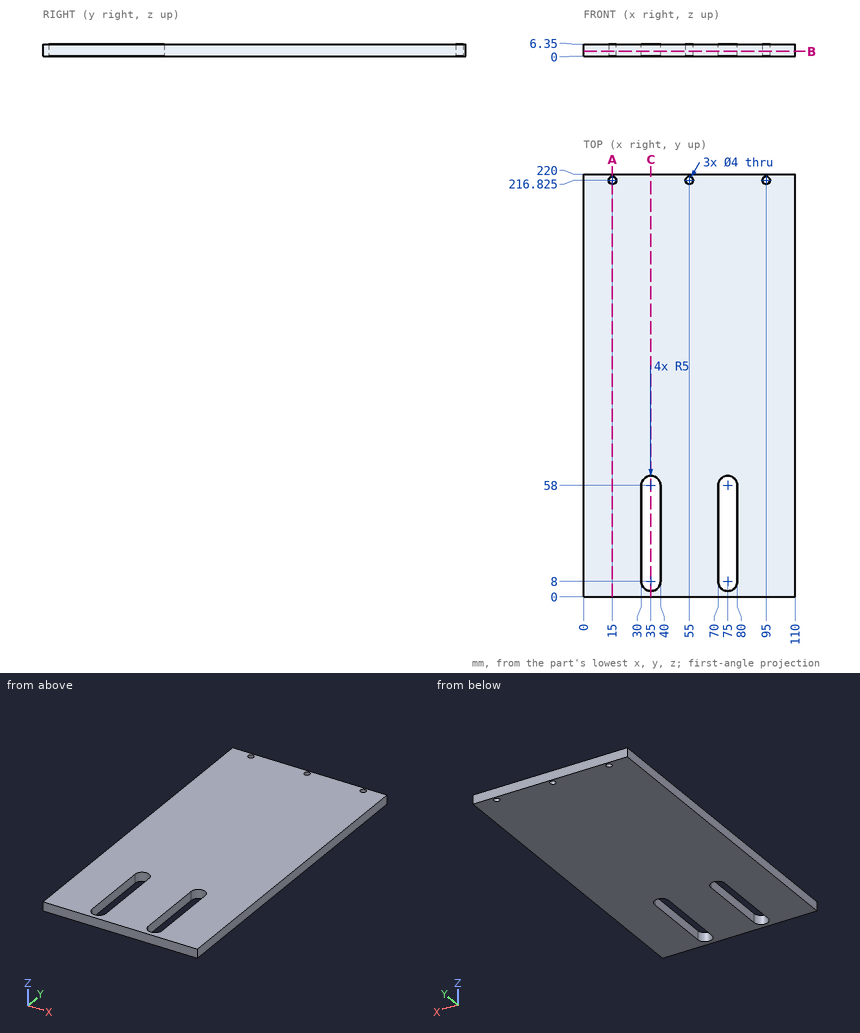
Input: dimensioned drawing with shaded views. Units: mm. Origin: part minimum x, y, z. Coordinates: 2 decimals unless noted, no trailing zeros. Write each loop counter-clockwise with the first axis right and the second up, starting at its lowest first coordinate (ties: lowest second). Pieces come first, ordered by that corner, then holes. Notation, with made-up numbers: (67, -34.75) -> (115, -34.75) arc R27 cw to (115, -4.75) -> close; hole circle Ø4 at (1, -3.75). An arc over 180 degrees is marked (long way). Return JSON: item names as keys, results as strings. Group by question number.
1) Ray query, line 1 along X through (y, z) = (31.5, 5.75); line 2 along Y through (x, z) = (15, 1.5) (3 decimals); line 3 along Y through (x, z) = (35, 2.75). Return the intervals inside material, ascending.
2) Section query B-B, the plane z = 2.5. Return loops of the section in (x, y) (3 decimals).
3) Contact query for a flat-ended pin moving along its axis: P1, Ø3, axis at x = 29.5, y = 85, coming from the -Z side. Output: stop coordinate, or through.
4) Section query C-C, the plane x = 35. Return loops of the section in (y, z), plus the area to 3 significant figures.
5) Section query A-A, the plane x = 15. Return loops of the section in (y, z) (3 decimals).
From the geometry:
{
 "1": {"line 1": "0 to 30, 40 to 70, 80 to 110", "line 2": "0 to 214.825, 218.825 to 220", "line 3": "0 to 3, 63 to 220"},
 "2": {"outline": "(0, 0) -> (110, 0) -> (110, 220) -> (0, 220) -> close; hole circle Ø4 at (15, 216.825); hole (30, 8) arc R5 ccw to (40, 8) -> (40, 58) arc R5 ccw to (30, 58) -> close; hole circle Ø4 at (55, 216.825); hole (70, 8) arc R5 ccw to (80, 8) -> (80, 58) arc R5 ccw to (70, 58) -> close; hole circle Ø4 at (95, 216.825)"},
 "3": {"P1": "z = 0"},
 "4": {"outline": "(0, 0) -> (3, 0) -> (3, 6.35) -> (0, 6.35) -> close; (63, 0) -> (220, 0) -> (220, 6.35) -> (63, 6.35) -> close", "area": "1,020 mm²"},
 "5": {"outline": "(0, 0) -> (214.825, 0) -> (214.825, 6.35) -> (0, 6.35) -> close; (218.825, 0) -> (220, 0) -> (220, 6.35) -> (218.825, 6.35) -> close"}
}
